```python
from build123d import *

# Parameters (mm, degrees)
SKETCH_1_R          = 2.518951354
EXTRUDE_1_DEPTH     = 5
SKETCH_2_R          = 5
CUT_EXTRUDE_1_DEPTH = 5


with BuildPart() as part:
    # 草图1 → 凸台-拉伸1 (new body)
    with BuildSketch(Plane.XY):
        with BuildLine():
            Line((0, 6), (50, 6))
            ThreePointArc((50, 6), (56, 0), (50, -6))
            Line((50, -6), (0, -6))
            ThreePointArc((0, -6), (-6, 0), (0, 6))
        make_face()
        with Locations((50, 0)):
            Circle(SKETCH_1_R, mode=Mode.SUBTRACT)
    extrude(amount=EXTRUDE_1_DEPTH)

    # 草图2 → 切除-拉伸1 (cut)
    with BuildSketch(Plane.XY.offset(5)):
        Circle(SKETCH_2_R)
    extrude(amount=-CUT_EXTRUDE_1_DEPTH, mode=Mode.SUBTRACT)


solid = part.part
```
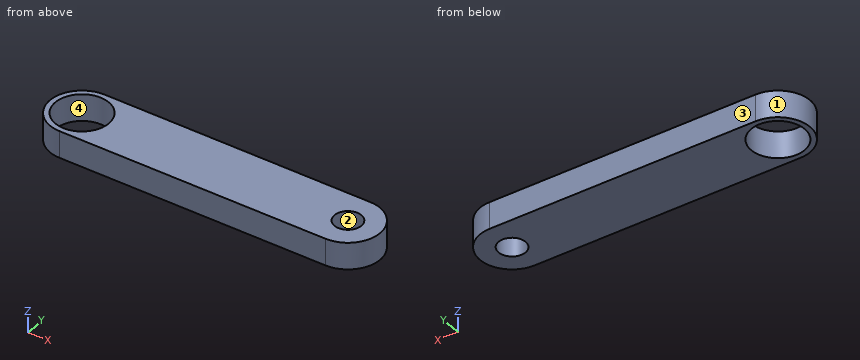
CAD build for the part. Positions are in the model's coordinates, mm. Face numbers are marked on the shaded views. Round coordinates to 2 decimals unless told otherwise and drop trailing zeros. Loops run counter-clockwise (first coordinate to the right, second up) from the corner with the lowest first, then second, coordinate; pieces in that order, holes last. Notation, with made-up numbers: (45, 6) - (59, 6) arc R13 ccw to (59, 25) - close; hole circle Ø7 at (67, -16). An arc over 180 degrees is marked (long way). Return JSON: item names as keys, results as strings. Group by question number.
Q1. Flat gauge pin, fed straight in: pin 1 Ø1 at (y, z) = (3.5, 3.5) entering from +X. Where does the tip first touch, or does it go through?
Q2. Band-saw the part on A-A on y = 0. Give the cut face in (x, z).
Q3. Drill centre lines: line 1 along X through (y, z) = (-0.25, 2.05); line 2 along Y through (x, z) = (50, 3.35); line 3 along Y through (x, z) = (0, 3.7). Where is each one in solid material? Low to high. Write a range as [from, to].
Q4. Band-saw the part on C-C on y = 3.5. Give the cut face in (x, z).
Q5. Two-plate mould, pull along Y, no slides. Class the marked faces 1, 2, 3 and 4: +Y half, -Y half, draft (parallel to the pull), parting line (faces both ways), or undercut.
Q6. Band-saw the part on B-B on z = 3.2. Give the cut face in (x, y).
Solutions:
{
 "1": {"pin 1": "stops at x = 55.2"},
 "2": {"outline": "(-6, 0) - (-5, 0) - (-5, 5) - (-6, 5) - close; (5, 0) - (47.48, 0) - (47.48, 5) - (5, 5) - close; (52.52, 0) - (56, 0) - (56, 5) - (52.52, 5) - close"},
 "3": {"line 1": "x = [-5.99, -4.99], [4.99, 47.49], [52.51, 55.99]", "line 2": "y = [-6, -2.52], [2.52, 6]", "line 3": "y = [-6, -5], [5, 6]"},
 "4": {"outline": "(-4.87, 0) - (-3.57, 0) - (-3.57, 5) - (-4.87, 5) - close; (3.57, 0) - (54.87, 0) - (54.87, 5) - (3.57, 5) - close"},
 "5": {"face 1": "parting line", "face 2": "undercut", "face 3": "+Y half", "face 4": "undercut"},
 "6": {"outline": "(0, -6) - (50, -6) arc R6 ccw to (50, 6) - (0, 6) arc R6 ccw to start; hole circle Ø10 at (0, 0); hole circle Ø5.04 at (50, 0)"}
}
